from build123d import *

# Parameters (mm, degrees)
SKETCH3_W           = 200
SKETCH3_H           = 10
BOSS_EXTRUDE1_DEPTH = 400
SKETCH4_R           = 5
BOSS_EXTRUDE2_DEPTH = 200
SKETCH5_W           = 180
SKETCH5_H           = 16
CUT_EXTRUDE1_DEPTH  = 75


with BuildPart() as part:
    # Sketch3 → Boss-Extrude1 (new body)
    with BuildSketch(Plane.XY):
        with Locations((100, 5)):
            Rectangle(SKETCH3_W, SKETCH3_H)
    extrude(amount=BOSS_EXTRUDE1_DEPTH)

    # Sketch4 → Boss-Extrude2 (add)
    with BuildSketch(Plane(origin=(200, 0, 0), x_dir=(0, 0, -1), z_dir=(1, 0, 0))):
        with BuildLine():
            Line((-342, 0), (-358, 0))
            Line((-358, 0), (-358, -9.403084831))
            Line((-358, -9.403084831), (-358, -10.596915169))
            ThreePointArc((-358, -10.596915169), (-350, -18.022238323), (-342, -10.596915169))
            Line((-342, -10.596915169), (-342, -9.403084831))
            Line((-342, -9.403084831), (-342, 0))
        make_face()
        with Locations((-350, -10)):
            Circle(SKETCH4_R, mode=Mode.SUBTRACT)
    extrude(amount=-BOSS_EXTRUDE2_DEPTH)

    # Sketch5 → Cut-Extrude1 (cut)
    with BuildSketch(Plane.XZ):
        with Locations((100, 350)):
            Rectangle(SKETCH5_W, SKETCH5_H)
    extrude(amount=CUT_EXTRUDE1_DEPTH, mode=Mode.SUBTRACT)


solid = part.part
Could you check a few things on this model? Use its own coordinates, in mm. A direction names the side the tool comes from. Give positions to 0.01 mm unless a question says otherwise; leave off trailing zeros. Write each loop counter-clockwise with the first axis right and the second up, starting at its lowest first coordinate (ties: lowest second). Pieces come first, ordered by that corner, then holes. Notation, with made-up numbers: (48.5, 17) - (81.5, 17) arc R22 ccw to (81.5, 44) - close; hole circle Ø8 at (20.25, -7). An arc over 180 degrees is marked (long way). Use CSV: the item, a comma, the result in double quotes. Start each with the question number.
Item 1: I'm going to push flat-ended pins straight in: pin 1 (16 mm diameter, centred on y = -10, z = 350, fed in from -X); pin 2 (5 mm diameter, centred on x = 196, y = -4.5, fed in from -Z); pin 3 (5 mm diameter, centred on x = 3.5, y = -5.5, fed in from +Z); pin 4 (10 mm diameter, centred on x = 45, z = 77, fed in from -Y). Where does each tip first touch, or does it pass through?
Item 2: If we mould it in two halves opening along X, with no side actions, what happens to faces 1 (the face through (99, 5, 0)), 2 (the face through (10, -5, 352)), 3 (the face through (0, 5, 214)), 4 (the face through (190, -5, 352))? For each: pulls with the +X half, pulls with the -X half, needs draft (parallel to the pull), parting line crosses it, or undercut.
Item 3: For faces 5 (the face through (195.07, -18.02, 350.17)), 6 (the face through (5, -5, 358)), 7 (the face through (5, -5, 342)), which set-ups out of +Z, -Z, +X, -X, +Y, -Y let a thin tool reach every point of the face, with its end or its side?
Item 4: If I drill on line 1 along Y through (x, z) = (2.5, 350); line 2 along Y through (x, z) = (186.5, 94.5); line 3 along Z through (x, y) = (191, -11.5), over which ranges is the centre line in solid material (lowest first)?
Item 5: I want a section at B-B, the plane x = 78. Please give me the cut outline in (y, z), then the cut area to 3 significant figures.
Item 6: I want a section at A-A, the plane z = 350. Please give me the cut outline in (x, y), then the cut area to 3 significant figures.
Findings:
1,pin 1,"stops at x = 0"
1,pin 2,"stops at z = 342"
1,pin 3,"stops at z = 358"
1,pin 4,"stops at y = 0"
2,face 1,"needs draft"
2,face 2,"undercut"
2,face 3,"pulls with the -X half"
2,face 4,"undercut"
3,face 5,"+X, -X, -Y"
3,face 6,"+Z, +X, -X, -Y"
3,face 7,"-Z, +X, -X, -Y"
4,line 1,"y = -18.02 to -15, -5 to 10"
4,line 2,"y = 0 to 10"
4,line 3,"z = 342.12 to 345.23, 354.77 to 357.88"
5,outline,"(0, 0) - (10, 0) - (10, 400) - (0, 400) - close"
5,area,"4,000 mm2"
6,outline,"(0, -18.02) - (10, -18.02) - (10, -15) - (0, -15) - close; (0, -5) - (10, -5) - (10, 0) - (190, 0) - (190, -5) - (200, -5) - (200, 10) - (0, 10) - close; (190, -18.02) - (200, -18.02) - (200, -15) - (190, -15) - close"
6,area,"2,160 mm2"
